Check sheet for the modelled part. Datum: model origin and axes. Units: mm. Face numbers are marked on the shaded views. A direction names the side the tool comes from. Give positions to 0.01 mm unless a question says otherwise; leave off trailing zeros. Loops run counter-clockwise (first coordinate to the right, second up) from the corner with the lowest first, then second, coordinate; pieces in that order, holes last. Notation, with made-up numbers: (81.5, -15.5) -> (128.5, -15.5) arc R19 ccw to (128.5, 4.5) -> close; hole circle Ø1 at (-19.75, 0). An arc over 180 degrees is marked (long way). Write each question's results on one line, items separated by ' | '. Start each with the question number.
1. Tool access check on the marked faces 1, 2 and 3. Record the directions out of +Z, -Z, +X, -X, +Y, -Y that give a thin tool (end or side, any length) a straight path to the whole face; none if there is none.
2. Gauge pin test, flat ends, axial feed: pin 1 Ø6 at (x, y) = (5.5, -38.5) entering from +Z; pin 2 Ø2 at (x, y) = (5.5, 7) entering from +Z; pin 3 Ø2 at (x, y) = (-6.5, 41.5) entering from -Z; pin 4 Ø12 at (x, y) = (-7, -48) entering from -Z. Record the tip position at first contact, or that the pin passes through.
3. Mould release check, pull along Y, two halves, no side actions. Record for the marked faces 4, 5 and 6: +Y half, -Y half, draft (parallel to the pull), parting line (faces both ways), or undercut.
4. Cross-section at C-C on z = 8.5. Record the boundary of the cut face in (x, y) (3 decimals).
5. Cross-section at D-D on z = 47. Record the boundary of the cut face in (x, y).
6. Material ranges on L1, parallel to Z at x = -3, y = -9; L2, parallel to Z at x = 0, y = 28.5; L3, parallel to Y at x = -0.5, z = 23, recorded low to high. Write a range as from..to.
7. Cross-section at B-B on x = 0. Record the boundary of the cut face in (y, z) (3 decimals), and give its area (3 significant figures).
8. Cross-section at A-A on y = 0. Record the boundary of the cut face in (x, z) (3 decimals), and give its area (3 significant figures).
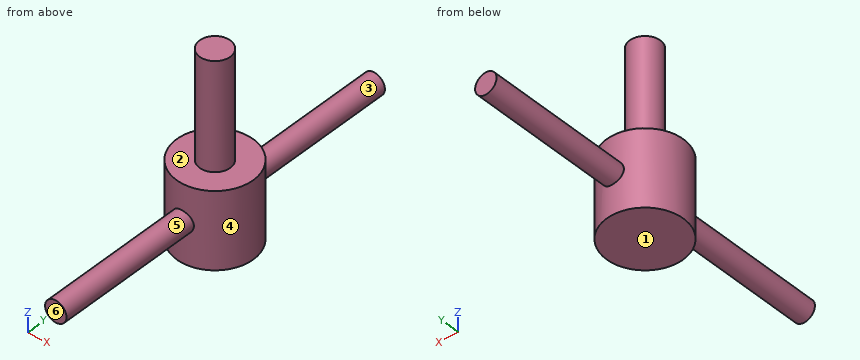
from build123d import *

# Parameters (mm, degrees)
F0_R     = 15.875
F1_DEPTH = 31.75
F2_R     = 6.35
F3_DEPTH = 44.45
F4_R     = 4.445
F5_DEPTH = 76.2


with BuildPart() as f1:
    # F0 (on Top) → F1 (new body)
    with BuildSketch(Plane.XY):
        Circle(F0_R)
    extrude(amount=F1_DEPTH)

    # F2 (on face) → F3 (join)
    with BuildSketch(Plane.XY.offset(31.75)):
        Circle(F2_R)
    extrude(amount=F3_DEPTH)

    # F4 (on Front) → F5 (join, symmetric)
    with BuildSketch(Plane.XZ):
        with Locations((0, 16.606679)):
            Circle(F4_R)
    extrude(amount=F5_DEPTH, both=True)


solid = f1.part
Geometry says:
1) face 1: -Z, +X, -X, +Y, -Y | face 2: +Z | face 3: +Y
2) pin 1: z = 20.28 | pin 2: z = 31.75 | pin 3: through | pin 4: z = 12.28
3) face 4: parting line | face 5: draft | face 6: -Y half
4) outline: circle Ø31.75 at (0, 0)
5) outline: circle Ø12.7 at (0, 0)
6) L1: 0..31.75 | L2: 12.16..21.05 | L3: -15.87..15.87
7) outline: (-76.2, 12.162) -> (-15.875, 12.162) -> (-15.875, 0) -> (15.875, 0) -> (15.875, 12.162) -> (76.2, 12.162) -> (76.2, 21.052) -> (15.875, 21.052) -> (15.875, 31.75) -> (6.35, 31.75) -> (6.35, 76.2) -> (-6.35, 76.2) -> (-6.35, 31.75) -> (-15.875, 31.75) -> (-15.875, 21.052) -> (-76.2, 21.052) -> close | area: 2,650 mm^2
8) outline: (-15.875, 0) -> (15.875, 0) -> (15.875, 31.75) -> (6.35, 31.75) -> (6.35, 76.2) -> (-6.35, 76.2) -> (-6.35, 31.75) -> (-15.875, 31.75) -> close | area: 1,570 mm^2
